Read the model definition and answer for the solid it produces. Units are mm, in the model's axes. A direction names the side the tool comes from. Give positions to 0.01 mm unless a question says otherwise; leave off trailing zeros. Loops run counter-clockwise (first coordinate to the right, second up) from the corner with the lowest first, then second, coordinate; pieces in that order, holes last. Notation, with made-up numbers: (-14, 1.25) - (-8, 1.25) arc R15 ccw to (-8, 30.25) - close; hole circle Ø6 at (61, -16). An arc over 180 degrees is marked (long way). Use a Markdown table: item, result. Add a question column.
Item 1: A cutting plane is placed at C-C (y = -23.5). Determine the outline of the cut face in (x, z), plus the area to 3 significant figures.
Item 2: Consider probe 1 along Y at (x, z) = (0.75, 5.75); probe 2 along X at (y, z) = (-16.75, 0); probe 3 along Z at (x, y) = (0, 2.1). Determine where each line is inside the solid, lowest interval first. Write a range as [from, to].
Item 3: Each of these flat-tipped pins is pushed along its axis until it touches: P1, Ø5, axis at x = -0.5, y = -17.5, coming from the -Z side; P2, Ø2.5, axis at x = 0, z = 0, coming from the +Y side; P3, Ø2.5, axis at x = 0, z = 5, coming from the +Y side; P4, Ø4, axis at x = 0, z = 0, coming from the +Y side. Where does it stop, or does it pass through?
Item 4: A cutting plane is placed at B-B (y = -1). Determine the outline of the cut face in (x, z).
Item 5: For a pull along X with two mould halves and no side action, classify faces 5 (the face through (-1.5, -37, 3)), 6 (the face through (0, -5, 4)), 7 (the face through (-5, -23, 3)), 8 (the face through (5, -23, 3)) as +X half, -X half, draft (parallel to the pull), parting line (faces both ways), or undercut.
Item 6: A cutting plane is placed at A-A (x = 0). Give the number of separate pieces and of enclosed holes in the cut face, plus the area to 3 significant figures.
Item 7: Which of the six approach directions +Z, -Z, +X, -X, +Y, -Y give full straight-line access (tool end or side, diameter ignored) to faces 1 (the face through (-1.5, -8, 3)), 2 (the face through (-0.1, -45, 3.4)), 3 (the face through (-0.1, 0, 3.4)), 4 (the face through (0, -23, 6.5))?
from build123d import *

# Parameters (mm, degrees)
F0_R     = 3
F0_R_2   = 1.5
F1_DEPTH = 22.5
F2_DEPTH = 10
F3_R     = 3
F3_R_2   = 1.5
F4_DEPTH = 5
F5_SIZE  = 1
F6_W     = 3
F6_H     = 6
F7_DEPTH = 6.5


with BuildPart() as f1:
    # F0 (on Front) → F1 (new body)
    with BuildSketch(Plane.XZ):
        with BuildLine():
            Line((5, 0), (5, 6.5))
            Line((5, 6.5), (-5, 6.5))
            Line((-5, 6.5), (-5, 1.3228756555))
            ThreePointArc((-5, 1.3228756555), (-4.5029510677, 0.1086073746), (-4.8653846154, -1.1524029436))
            ThreePointArc((-4.8653846154, -1.1524029436), (-4.8296291314, -1.2940952255), (-4.7897481479, -1.4346820832))
            ThreePointArc((-4.7897481479, -1.4346820832), (-3.897114317, -2.25), (-3.6373452043, -3.4307025322))
            ThreePointArc((-3.6373452043, -3.4307025322), (-3.5355339059, -3.5355339059), (-3.4307025322, -3.6373452043))
            ThreePointArc((-3.4307025322, -3.6373452043), (-2.25, -3.897114317), (-1.4346820832, -4.7897481479))
            ThreePointArc((-1.4346820832, -4.7897481479), (-1.2940952255, -4.8296291314), (-1.1524029436, -4.8653846154))
            ThreePointArc((-1.1524029436, -4.8653846154), (0, -4.5), (1.1524029436, -4.8653846154))
            ThreePointArc((1.1524029436, -4.8653846154), (3.921862741, -3.1014500868), (5, 0))
        make_face()
        Circle(F0_R, mode=Mode.SUBTRACT)
        Circle(F0_R)
        Circle(F0_R_2, mode=Mode.SUBTRACT)
    extrude(amount=F1_DEPTH)

    # F0 (on Front) → F2 (join)
    with BuildSketch(Plane.XZ):
        with BuildLine():
            ThreePointArc((-4.8653846154, -1.1524029436), (-4.5029510677, 0.1086073746), (-5, 1.3228756555))
            Line((-5, 1.3228756555), (-5, 0))
            ThreePointArc((-5, 0), (-4.9662321269, -0.5801193511), (-4.8653846154, -1.1524029436))
        make_face()
        with BuildLine():
            ThreePointArc((-3.6373452043, -3.4307025322), (-3.897114317, -2.25), (-4.7897481479, -1.4346820832))
            ThreePointArc((-4.7897481479, -1.4346820832), (-4.3301270189, -2.5), (-3.6373452043, -3.4307025322))
        make_face()
        with BuildLine():
            ThreePointArc((-3.4307025322, -3.6373452043), (-2.5, -4.3301270189), (-1.4346820832, -4.7897481479))
            ThreePointArc((-1.4346820832, -4.7897481479), (-2.25, -3.897114317), (-3.4307025322, -3.6373452043))
        make_face()
        with BuildLine():
            ThreePointArc((-1.1524029436, -4.8653846154), (0, -5), (1.1524029436, -4.8653846154))
            ThreePointArc((1.1524029436, -4.8653846154), (0, -4.5), (-1.1524029436, -4.8653846154))
        make_face()
    extrude(amount=F2_DEPTH)

    # F3 (on face) → F4 (join)
    with BuildSketch(Plane.XZ):
        Circle(F3_R)
        Circle(F3_R_2, mode=Mode.SUBTRACT)
    extrude(amount=-F4_DEPTH)

    # F5
    f5_edges = [f1.edges().sort_by_distance(p)[0] for p in [
        (-3, 5, 0),
    ]]
    chamfer(f5_edges, length=F5_SIZE)

    # F6 (on face) → F7 (cut, through all)
    with BuildSketch(Plane.XY.offset(6.5)):
        with Locations((0, -8)):
            Rectangle(F6_W, F6_H)
    extrude(amount=-F7_DEPTH, mode=Mode.SUBTRACT)

    # F8: F1 across face


with BuildPart() as f1_1:
    add(f1.part)
    add(f1.part.mirror(Plane(origin=(0.0969972457, -22.5, 1.4535836906), x_dir=(1, 0, 0), z_dir=(0, -1, 0))))


solid = f1_1.part
Geometry says:
| question | item | result |
|---|---|---|
| 1 | outline | (-5, 1.32) arc R2 cw to (-4.87, -1.15) arc R5 ccw to (-4.79, -1.43) arc R2 cw to (-3.64, -3.43) arc R5 ccw to (-3.43, -3.64) arc R2 cw to (-1.43, -4.79) arc R5 ccw to (-1.15, -4.87) arc R2 cw to (1.15, -4.87) arc R5 ccw to (5, 0) - (5, 6.5) - (-5, 6.5) - close; hole circle Ø3 at (0, 0) |
| 1 | area | 94.0 mm² |
| 2 | probe 1 | [-45, -40], [-34, -11], [-5, 0] |
| 2 | probe 2 | [-4.5, -1.5], [1.5, 5] |
| 2 | probe 3 | [-3, -1.5], [1.5, 3] |
| 3 | P1 | z = -4.87 |
| 3 | P2 | through |
| 3 | P3 | y = 0 |
| 3 | P4 | y = 5 |
| 4 | outline | (-5, 0) arc R5 ccw to (5, 0) - (5, 6.5) - (-5, 6.5) - close; hole circle Ø3 at (0, 0) |
| 5 | face 5 | undercut |
| 5 | face 6 | undercut |
| 5 | face 7 | -X half |
| 5 | face 8 | +X half |
| 6 | separate pieces | 4 |
| 6 | enclosed holes | 0 |
| 6 | area | 338 mm² |
| 7 | face 1 | +Z |
| 7 | face 2 | -Y |
| 7 | face 3 | +Y |
| 7 | face 4 | +Z, +X, -X, +Y, -Y |
